from build123d import *

# Parameters (mm, degrees)
SKETCH_1_W             = 16
SKETCH_1_H             = 57
EXTRUDE_1_DEPTH        = 6
SKETCH_2_W             = 31.720899854
SKETCH_2_H             = 10
CUT_EXTRUDE_1_DEPTH    = 1
SKETCH_3_W             = 4
SKETCH_3_H             = 5
EXTRUDE_2_DEPTH        = 6
HOLE_WIZARD_M3_1_D     = 2.5
HOLE_WIZARD_M3_1_DEPTH = 7.5
HOLE_WIZARD_M3_1_TIP   = 0.751075774
SKETCH_6_W             = 7
SKETCH_6_H             = 1
CUT_EXTRUDE_2_DEPTH    = 58
SKETCH_7_R             = 2.25
CUT_EXTRUDE_3_DEPTH    = 6


with BuildPart() as part:
    # 草图1 → 凸台-拉伸1 (new body)
    with BuildSketch(Plane.XY):
        with Locations((8, 28.5)):
            Rectangle(SKETCH_1_W, SKETCH_1_H)
    extrude(amount=EXTRUDE_1_DEPTH)

    # 草图2 → 切除-拉伸1 (cut)
    with BuildSketch(Plane.XY.offset(6)):
        with Locations((15.860449927, 52)):
            Rectangle(SKETCH_2_W, SKETCH_2_H)
    extrude(amount=-CUT_EXTRUDE_1_DEPTH, mode=Mode.SUBTRACT)

    # 草图3 → 凸台-拉伸2 (add)
    with BuildSketch(Plane(origin=(0, 0, 0), x_dir=(-1, 0, 0), z_dir=(0, 0, -1))):
        with Locations((-18, 22.6)):
            Rectangle(SKETCH_3_W, SKETCH_3_H)
        with Locations((2, 22.6)):
            Rectangle(SKETCH_3_W, SKETCH_3_H)
    extrude(amount=-EXTRUDE_2_DEPTH)

    # M3 螺纹孔1
    with Locations(Plane(origin=(0, 0, 0), x_dir=(-1, 0, 0), z_dir=(0, 0, -1))):
        with Locations((-8, 35), (-8, 20), (-8, 5)):
            Hole(HOLE_WIZARD_M3_1_D / 2, depth=HOLE_WIZARD_M3_1_DEPTH)
            with Locations((0, 0, -(HOLE_WIZARD_M3_1_DEPTH + HOLE_WIZARD_M3_1_TIP / 2))):  # 118° drill point
                Cone(0, HOLE_WIZARD_M3_1_D / 2, HOLE_WIZARD_M3_1_TIP, mode=Mode.SUBTRACT)

    # 草图6 → 切除-拉伸2 (cut, through all)
    with BuildSketch(Plane.XZ):
        with Locations((8, 5.5)):
            Rectangle(SKETCH_6_W, SKETCH_6_H)
    extrude(amount=-CUT_EXTRUDE_2_DEPTH, mode=Mode.SUBTRACT)

    # 草图7 → 切除-拉伸3 (cut, through all)
    with BuildSketch(Plane.XY.offset(5)):
        with Locations((3.25, 52)):
            Circle(SKETCH_7_R)
        with Locations((12.75, 52)):
            Circle(SKETCH_7_R)
    extrude(amount=-CUT_EXTRUDE_3_DEPTH, mode=Mode.SUBTRACT)


solid = part.part
Geometry: final body of the model. Coordinates: model frame, mm. A direction names the side the tool comes from. Give positions to 0.01 mm unless a question says otherwise; leave off trailing zeros. Loops run counter-clockwise (first coordinate to the right, second up) from the corner with the lowest first, then second, coordinate; pieces in that order, holes last. Notation, with made-up numbers: M 44.25,85.5 L 54.25,85.5 A9 cw 54.25,97.5 Z; hole C 43.5,-32 d9. An arc over 180 degrees is marked long. Put each result on its own line as item: value. Start each with the question number.
1) Ray query, line 1 along Y through (x, z) = (8, 1.45); line 2 along Y through (x, z) = (3.25, 1.4); line 3 along X through (y, z) = (25.5, 5.5). Return the intervals inside material, ascending.
2) Contact query for flat-ended pins moving along their axis: pin 1 (2 mm diameter, centred on x = 8, y = 35, fed in from +Z); pin 2 (2 mm diameter, centred on x = 17.5, z = 1.5, fed in from +Y); pin 3 (1.8 mm diameter, centred on y = 36.5, z = 2, fed in from -X); pin 4 (3 mm diameter, centred on x = 18, z = 4.5, fed in from -Y). Output: stop coordinate, or through.
3) Access query for faces 1 (the flat face through (0, 41, 3)), 2 (the flat face through (0, 10, 3)), 3 (the flat face through (13.7, 47, 5.5)), 4 (the flat face through (4.5, 23.2, 5.5)). Directions: +Z, -Z, +X, -X, +Y, -Y. A direction counts if a zero-diameter tool reaches every point of the face in a straight line with its end or side. Return the directions, or none.
4) Cut plane A-A (y = 5). Output: boundary loops of the cut face in (x, z), then the cut area to 3 significant figures.
5) Cut plane D-D (x = 3.25). Output: boundary loops of the cut face in (y, z), then the cut area to 4 significant figures.
6) Cut plane B-B (x = 8.75). Output: boundary loops of the cut face in (y, z).
7) Cut plane C-C (y = 52). Output: boundary loops of the cut face in (x, z), then the cut area to 3 significant figures.
8) Pull-direction query (Y, two-part tool) for faces 5 (the flat face through (8, 0, 3)), 6 (the cylindrical face through (7.01, 4.24, 2.54)), 7 (the flat face through (20, 23, 3)), 8 (the flat face through (-2, 25.1, 3)); classes: pulls with the +Y half, pulls with the -Y half, needs draft (parallel to the pull), parting line crosses it, or undercut.
Verdict:
1. line 1: 0 to 3.75, 6.25 to 18.75, 21.25 to 33.75, 36.25 to 57
1. line 2: 0 to 49.75, 54.25 to 57
1. line 3: 0 to 4.5, 11.5 to 16
2. pin 1: through
2. pin 2: y = 25.1
2. pin 3: x = 0
2. pin 4: y = 20.1
3. face 1: +Z, -Z, -X, +Y
3. face 2: +Z, -Z, -X, -Y
3. face 3: +Z, +X, -X, +Y
3. face 4: +Z, +Y, -Y
4. outline: M 0,0 L 6.75,0 L 6.75,5 L 4.5,5 L 4.5,6 L 0,6 Z; M 9.25,0 L 16,0 L 16,6 L 11.5,6 L 11.5,5 L 9.25,5 Z
4. area: 76.5 mm2
5. outline: M 0,0 L 49.75,0 L 49.75,5 L 47,5 L 47,6 L 0,6 Z; M 54.25,0 L 57,0 L 57,5 L 54.25,5 Z
5. area: 309.5 mm2
6. outline: M 0,0 L 4,0 L 4,5 L 0,5 Z; M 6,0 L 19,0 L 19,5 L 6,5 Z; M 21,0 L 34,0 L 34,5 L 21,5 Z; M 36,0 L 57,0 L 57,5 L 36,5 Z
7. outline: M 0,0 L 1,0 L 1,5 L 0,5 Z; M 5.5,0 L 10.5,0 L 10.5,5 L 5.5,5 Z; M 15,0 L 16,0 L 16,5 L 15,5 Z
7. area: 35.0 mm2
8. face 5: pulls with the -Y half
8. face 6: undercut
8. face 7: needs draft
8. face 8: pulls with the +Y half
